Build history of the part. All positions in model axes, mm. A direction names the side the tool comes from. Give positions to 0.01 mm unless a question says otherwise; leave off trailing zeros. Order: outer loops, then holes, each group sorted by start corner. A loop starts at its lowest first (then second) coordinate and runs counter-clockwise, first axis right, second up. Notation, with made-up numbers: (32.25, 82.5) - (36.25, 82.5) arc R15 cw to (36.25, 91.5) - close; hole circle Ø9 at (82, 12.25). An arc over 180 degrees is marked (long way). One line per item, written item: value.
```python
from build123d import *

# Parameters (mm, degrees)
F0_W        = 28.7667152895
F0_H        = 25.4
F0_R        = 1.7375
F0_R_2      = 3.96875
F1_DEPTH    = 5.08
F2_W        = 35.1060024381
F2_H        = 33.9911315718
F2_R        = 12.5
F3_DEPTH    = 35
F4_T1_DEPTH = 59.3911315718
F4_T3_DEPTH = 95.4


# Not quite as in the source:
# - a fillet or chamfer that OpenCascade refuses, or shapes differently, is made with other operations: its cross-section is extruded or revolved along the edge and cut away or added
# - a feature names something its author has since deleted; it is built from what else it names


with BuildPart() as f1:
    # F0 (on Top) → F1 (new body)
    with BuildSketch(Plane.XY):
        with Locations((28.4760861403, 0)):
            Rectangle(F0_W, F0_H)
        with Locations((29.5036397874, -8.8014880077)):
            Circle(F0_R, mode=Mode.SUBTRACT)
        with Locations((20.6223897874, 0.0797619923)):
            Circle(F0_R, mode=Mode.SUBTRACT)
        with Locations((29.5036397874, 0.0797619923)):
            Circle(F0_R_2, mode=Mode.SUBTRACT)
        with Locations((38.3848897874, 0.0797619923)):
            Circle(F0_R, mode=Mode.SUBTRACT)
        with Locations((29.5036397874, 8.9610119923)):
            Circle(F0_R, mode=Mode.SUBTRACT)
    extrude(amount=F1_DEPTH)

    # F2 (on Top) → F3 (join, symmetric)
    with BuildSketch(Plane.XY):
        with Locations((-1.2872326612, 0)):
            Rectangle(F2_W, F2_H)
        with Locations((-1.4946922893, 0)):
            Circle(F2_R, mode=Mode.SUBTRACT)
    extrude(amount=F3_DEPTH, both=True)

    # F4: fillet of radius 5.08 on 3 edges, made by hand

    # F4_s2 → F4_t1 (cut)
    with BuildSketch(Plane.XZ.offset(-29.6955657859)):
        with BuildLine():
            ThreePointArc((-13.7602338803, 35), (-17.3523363287, 33.5121024484), (-18.8402338803, 29.92))
            Line((-18.8402338803, 29.92), (-18.8402338803, 35))
            Line((-18.8402338803, 35), (-13.7602338803, 35))
        make_face()
    extrude(amount=F4_T1_DEPTH, mode=Mode.SUBTRACT)

    # F4_s4 → F4_t3 (cut)
    with BuildSketch(Plane.XY.offset(-47.7)):
        with BuildLine():
            ThreePointArc((-13.7602338803, -16.9955657859), (-17.3523363287, -15.5076682343), (-18.8402338803, -11.9155657859))
            Line((-18.8402338803, -11.9155657859), (-18.8402338803, -16.9955657859))
            Line((-18.8402338803, -16.9955657859), (-13.7602338803, -16.9955657859))
        make_face()
        with BuildLine():
            ThreePointArc((-13.7602338803, 16.9955657859), (-17.3523363287, 15.5076682343), (-18.8402338803, 11.9155657859))
            Line((-18.8402338803, 11.9155657859), (-18.8402338803, 16.9955657859))
            Line((-18.8402338803, 16.9955657859), (-13.7602338803, 16.9955657859))
        make_face()
    extrude(amount=F4_T3_DEPTH, mode=Mode.SUBTRACT)


solid = f1.part
```
(1) Pin check, flat tips, straight feed: P1, Ø4.5, axis at x = 29.5, y = 8.96, coming from the -Z side; P2, Ø6, axis at x = 34, z = 9, coming from the +Y side; P3, Ø4, axis at x = 35.5, z = 4, coming from the -Y side; P4, Ø4, axis at y = 4, z = -2.5, coming from the +X side. Stop position of each tip, or through.
Completed:
P1: z = 0
P2: through
P3: y = -12.7
P4: x = 16.27
(2) Pull direction X, two halves, no side cores. Call faces 1 (the face through (28.22, -7.63, 2.5)), 2 (the face through (25.54, 0.25, 2.5)), 3 (the face through (-9, 12, -35)), 4 (the face through (-17.313, 0.238, 33.551)): +X half, -X half, draft (parallel to the pull), parting line (faces both ways), or undercut.
Completed:
face 1: undercut
face 2: undercut
face 3: draft
face 4: -X half
(3) Slice it at C-C, the plane y = -14.5. Give the cut face in (x, z).
Completed:
outline: (-18.13, -35) - (16.27, -35) - (16.27, 35) - (-13.76, 35) arc R5.08 ccw to (-18.13, 32.5) - close
(4) Slice it at B-B, the plane z = 7. Give the cut face in (x, y), and give its area (3 significant figures).
Completed:
outline: (-18.84, -11.92) arc R5.08 ccw to (-13.76, -17) - (16.27, -17) - (16.27, 17) - (-13.76, 17) arc R5.08 ccw to (-18.84, 11.92) - close; hole circle Ø25 at (-1.49, 0)
area: 691 mm²
(5) 3-axis set-ups, long thin cutter, end or side, ignore diameter. For faces 5 (the face through (26, 3, 5.08)), 6 (the face through (26, 3, 0)), 7 (the face through (29, -12.7, 3)), 8 (the face through (29, 12.7, 3)): which of +Z, -Z, +X, -X, +Y, -Y reach the whole face in a straight line?
Completed:
face 5: +Z, +X, +Y, -Y
face 6: -Z, +X, +Y, -Y
face 7: +Z, -Z, +X, -Y
face 8: +Z, -Z, +X, +Y
(6) Drill centre lines: line 1 (X direction, y = 0, z = -4); line 2 (Y direction, x = 3, z = 0); line 3 (Z direction, x = 37, y = 7). Where is each one in solid material? Low to high.
Completed:
line 1: -18.84 to -13.99, 11.01 to 16.27
line 2: -17 to -11.66, 11.66 to 17
line 3: 0 to 5.08
(7) Slice it at A-A, the plane x = -1.5. Give the cut face in (y, z), and give its area (3 significant figures).
Completed:
outline: (-17, -35) - (-12.5, -35) - (-12.5, 35) - (-17, 35) - close; (12.5, -35) - (17, -35) - (17, 35) - (12.5, 35) - close
area: 629 mm²
